CAD build for the part. Positions are in the model's coordinates, mm. Coordinates: 2 decimals unless noted, no trailing zeros. Write each loop counter-clockwise with the first axis right and the second up, starting at its lowest first coordinate (ties: lowest second). Pieces come first, ordered by that corner, then holes. Notation, with made-up numbers: (45.25, 31) - (100.25, 31) arc R19 ccw to (100.25, 49) - close; hole circle Ø9 at (-23, 54). An arc over 180 degrees is marked (long way). One line per question, with ' | ' between items. Start each with the question number.
1. Band-saw the part on B-B, the plane y = -8.5. Write the cut outline in (x, z), then the cut area to 3 significant figures.
2. Flat gauge pins, fed straight in: P1, Ø4, axis at x = 45, z = 0.5, coming from the +Y side; P2, Ø4, axis at y = -149.5, z = 23, coming from the -X side; P3, Ø6, axis at x = 196, y = -74.5, coming from the +Z side. Where does each tip first touch, or does it go through?
3. Band-saw the part on A-A, the plane y = -137. Write the cut outline in (x, z), then the cut area to 3 significant figures.
4. Band-saw the part on D-D, the plane y = -54. Write the cut outline in (x, z).
5. Band-saw the part on C-C, the plane z = -8. Write the cut outline in (x, y), then the cut area to 3 significant figures.
6. Probe line 1 (X direction, y = -126.5, z = -15.5); line 2 (Y direction, x = 165, z = 9); line 3 (Z direction, x = 68, y = -9). List the from-to ranges inside material, lowest first.
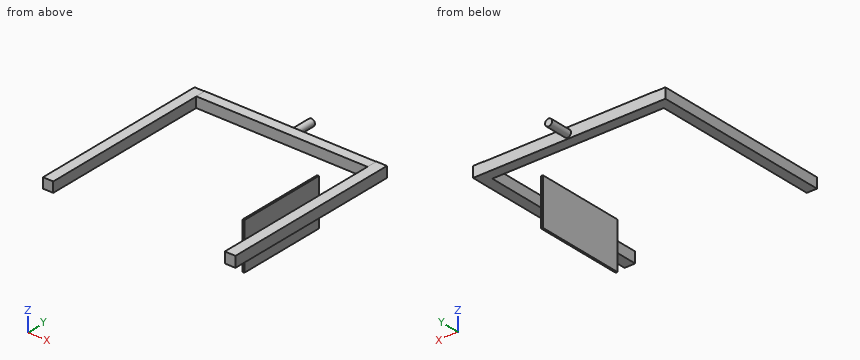
from build123d import *

# Parameters (mm, degrees)
F0_W     = 11.43
F0_H     = 11.285316
F1_DEPTH = 203.2
F2_W     = 11.558608
F2_H     = 11.574684
F3_DEPTH = 203.2
F4_W     = 11.864051
F4_H     = 11.86405
F5_DEPTH = 203.2
F6_W     = 99.82273
F6_H     = 51.891416
F7_DEPTH = 2.032
F8_R     = 3.935821
F9_DEPTH = 25.4


with BuildPart() as f1:
    # F0 (on Front) → F1 (new body)
    with BuildSketch(Plane.XZ):
        with Locations((-5.715, 5.642658)):
            Rectangle(F0_W, F0_H)
    extrude(amount=F1_DEPTH)

    # F2 (on Right) → F3 (join)
    with BuildSketch(Plane.YZ):
        with Locations((-5.779304, 5.787342)):
            Rectangle(F2_W, F2_H)
    extrude(amount=F3_DEPTH)

    # F4 (on Front) → F5 (join)
    with BuildSketch(Plane.XZ):
        with Locations((197.47696, 5.932025)):
            Rectangle(F4_W, F4_H)
    extrude(amount=F5_DEPTH)

    # F6 (on face) → F7 (join)
    with BuildSketch(Plane(origin=(191.544935, 0, 0), x_dir=(0, -1, 0), z_dir=(-1, 0, 0))):
        with Locations((126.978308, 5.327698)):
            Rectangle(F6_W, F6_H)
    extrude(amount=F7_DEPTH)

    # F8 (on face) → F9 (join)
    with BuildSketch(Plane(origin=(0, 0, 0), x_dir=(-1, 0, 0), z_dir=(0, 1, 0))):
        with Locations((-97.89449, 5.208607)):
            Circle(F8_R)
    extrude(amount=F9_DEPTH)


solid = f1.part
Filled in:
1) outline: (-11.43, 0) - (203.41, 0) - (203.41, 11.86) - (191.54, 11.86) - (191.54, 11.57) - (0, 11.57) - (0, 11.29) - (-11.43, 11.29) - close | area: 2,490 mm²
2) P1: stops at y = 0 | P2: stops at x = 189.51 | P3: stops at z = 11.86
3) outline: (-11.43, 0) - (0, 0) - (0, 11.29) - (-11.43, 11.29) - close; (189.51, -20.62) - (191.54, -20.62) - (191.54, 0) - (203.41, 0) - (203.41, 11.86) - (191.54, 11.86) - (191.54, 31.27) - (189.51, 31.27) - close | area: 375 mm²
4) outline: (-11.43, 0) - (0, 0) - (0, 11.29) - (-11.43, 11.29) - close; (191.54, 0) - (203.41, 0) - (203.41, 11.86) - (191.54, 11.86) - close
5) outline: (189.51, -176.89) - (191.54, -176.89) - (191.54, -77.07) - (189.51, -77.07) - close | area: 203 mm²
6) line 1: x = 189.51 to 191.54 | line 2: y = -11.56 to 0 | line 3: z = 0 to 11.57
